Check sheet for the modelled part. Datum: model origin and axes. Units: mm. Face numbers are marked on the shaded views. A direction names the side the tool comes from. Coordinates: 2 decimals unless noted, no trailing zeros. Write each loop counter-clockwise with the first axis right and the second up, starting at its lowest first coordinate (ties: lowest second). Pieces come first, ordered by that corner, then holes. Notation, with made-up numbers: (20, 78.5) - (71, 78.5) arc R24 cw to (71, 102.5) - close; hole circle Ø9 at (73.5, 87). An arc over 180 degrees is marked (long way). Use one line per item in the form item = value. Start each with the question number.
1. Cross-section at D-D on y = 6.5. Record the boundary of the cut face in (x, z).
2. Cross-section at A-A on y = 0. Record the boundary of the cut face in (x, z), then the cut area to 3 significant figures.
3. Scan lines: line 1 along Z through (x, y) = (0, -19.3); line 2 along X through (y, z) = (10, -5.25); line 3 along X through (y, z) = (-10.5, -6.75). Record each from-to range of solid material in increasing order.
4. Tool access check on the marked faces 5, 6 and 7. Record the directions out of +Z, -Z, +X, -X, +Y, -Y that give a thin tool (end or side, any length) a straight path to the whole face; none if there is none.
5. Go/stop test with flat-tipped pins: pin 1 Ø7 at (y, z) = (0, -5) entering from +X; pin 2 Ø2.5 at (x, z) = (1.5, -6.5) entering from +Y; pin 3 Ø2 at (y, z) = (16, -6) entering from -X. Record where each tip stops, or that it passes through.
6. Draft check along Z on the marked faces 1, 2, 3 and 4. Enter one of: +Z half, -Z half, draft (parallel to the pull), parting line (faces both ways), or undercut.
```python
from build123d import *

# Parameters (mm, degrees)
SKETCH3_R                 = 22.5
BOSS_EXTRUDE3_DEPTH       = 14.2
SKETCH8_R                 = 4
CUT_EXTRUDE4_DEPTH        = 5.5
SKETCH6_R                 = 2.75
CUT_EXTRUDE6_DEPTH        = 14.2
CIRPATTERN1_COUNT         = 8
SKETCH5_R                 = 8.1
CUT_EXTRUDE7_DEPTH        = 5.5
BOUNDARY_CUT1_START       = -12.2
BOUNDARY_CUT1_OUTLINE_R   = 22.5
BOUNDARY_CUT1_OUTLINE_R_2 = 22
BOUNDARY_CUT1_DEPTH       = 0.2


# Read off the part's stored shape, not the designer's step: Boundary-Cut1
with BuildPart() as part:
    # Sketch3 → Boss-Extrude3 (new body)
    with BuildSketch(Plane.XY):
        Circle(SKETCH3_R)
    extrude(amount=-BOSS_EXTRUDE3_DEPTH)

    # Sketch8 → Cut-Extrude4 (cut)
    with BuildSketch(Plane(origin=(22.5, 0, 0), x_dir=(0, 0, -1), z_dir=(1, 0, 0))):
        with Locations((5, 0)):
            Circle(SKETCH8_R)
    cut_extrude4 = extrude(amount=-CUT_EXTRUDE4_DEPTH, mode=Mode.SUBTRACT)

    # Sketch6 → Cut-Extrude6 (cut)
    with BuildSketch(Plane.XY):
        Circle(SKETCH6_R)
    extrude(amount=-CUT_EXTRUDE6_DEPTH, mode=Mode.SUBTRACT)

    # CirPattern1: Cut-Extrude4 ×8 about axis
    cirpattern1_axis = Axis((0, 0, 0), (0, 0, 1))
    for i in range(1, CIRPATTERN1_COUNT):
        add(cut_extrude4.rotate(cirpattern1_axis, i * 360 / CIRPATTERN1_COUNT), mode=Mode.SUBTRACT)

    # Sketch5 → Cut-Extrude7 (cut)
    with BuildSketch(Plane.XY):
        Circle(SKETCH5_R)
    extrude(amount=-CUT_EXTRUDE7_DEPTH, mode=Mode.SUBTRACT)

    # Boundary-Cut1 outline → Boundary-Cut1 (cut)
    with BuildSketch(Plane.XY.offset(BOUNDARY_CUT1_START)):
        Circle(BOUNDARY_CUT1_OUTLINE_R)
        Circle(BOUNDARY_CUT1_OUTLINE_R_2, mode=Mode.SUBTRACT)
    extrude(amount=BOUNDARY_CUT1_DEPTH, mode=Mode.SUBTRACT)


solid = part.part
```
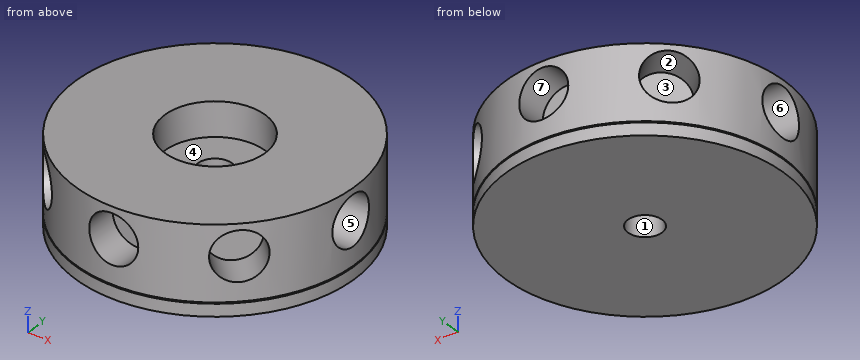
Final values:
q1.outline = (-21.54, -14.2) - (21.54, -14.2) - (21.54, -12.2) - (21.02, -12.2) - (21.02, -12) - (21.54, -12) - (21.54, 0) - (4.83, 0) - (4.83, -5.5) - (-4.83, -5.5) - (-4.83, 0) - (-21.54, 0) - (-21.54, -12) - (-21.02, -12) - (-21.02, -12.2) - (-21.54, -12.2) - close
q2.outline = (-22.5, -14.2) - (-2.75, -14.2) - (-2.75, -5.5) - (-8.1, -5.5) - (-8.1, 0) - (-22.5, 0) - (-22.5, -1) - (-17, -1) - (-17, -9) - (-22.5, -9) - (-22.5, -12) - (-22, -12) - (-22, -12.2) - (-22.5, -12.2) - close; (2.75, -14.2) - (22.5, -14.2) - (22.5, -12.2) - (22, -12.2) - (22, -12) - (22.5, -12) - (22.5, -9) - (17, -9) - (17, -1) - (22.5, -1) - (22.5, 0) - (8.1, 0) - (8.1, -5.5) - (2.75, -5.5) - close
q2.area = 414 mm²
q3.line_1 = -14.2 to -9, -1 to 0
q3.line_2 = -20.16 to -15.65, -14.04 to 14.04, 15.65 to 20.16
q3.line_3 = -19.9 to -15.59, -13.54 to 13.54, 15.59 to 19.9
q4.face_5 = +X
q4.face_6 = -X
q4.face_7 = +Y
q5.pin_1 = 17
q5.pin_2 = 17
q5.pin_3 = -11.62
q6.face_1 = draft
q6.face_2 = undercut
q6.face_3 = undercut
q6.face_4 = +Z half
